Part model, mm, in its own coordinate system. A direction names the side the tool comes from. Coordinates: 2 decimals unless noted, no trailing zeros. Loops run counter-clockwise (first coordinate to the right, second up) from the corner with the lowest first, then second, coordinate; pieces in that order, holes last. Notation, with made-up numbers: (69, 70.25) -> (122, 70.25) arc R34 cw to (122, 108.25) -> close; hole circle Ø9 at (43.25, 68.5). An arc over 180 degrees is marked (long way). One line per item, written item: value. Start each with the question number.
from build123d import *

# Parameters (mm, degrees)
SKETCH1_W               = 16
SKETCH1_H               = 24
BOSS_EXTRUDE1_DEPTH     = 1
SKETCH2_W               = 12.3
SKETCH2_H               = 15.2
BOSS_EXTRUDE2_DEPTH     = 2.4
SKETCH3_R               = 0.3
CUT_EXTRUDE1_DEPTH      = 15.817557154
LPATTERN1_COUNT         = 8
LPATTERN1_PITCH         = 2
MIRROR1_COPY_1_SKETCH_R = 0.3
MIRROR1_COPY_1_DEPTH    = 15.817557154
MIRROR1_COPY_2_SKETCH_R = 0.3
MIRROR1_COPY_2_DEPTH    = 15.817557154
MIRROR1_COPY_3_SKETCH_R = 0.3
MIRROR1_COPY_3_DEPTH    = 15.817557154
MIRROR1_COPY_4_SKETCH_R = 0.3
MIRROR1_COPY_4_DEPTH    = 15.817557154
MIRROR1_COPY_5_SKETCH_R = 0.3
MIRROR1_COPY_5_DEPTH    = 15.817557154
MIRROR1_COPY_6_SKETCH_R = 0.3
MIRROR1_COPY_6_DEPTH    = 15.817557154
MIRROR1_COPY_7_SKETCH_R = 0.3
MIRROR1_COPY_7_DEPTH    = 15.817557154
SKETCH4_R               = 0.3
CUT_EXTRUDE2_DEPTH      = 15.817557154
LPATTERN2_COUNT         = 6
LPATTERN2_PITCH         = 2


with BuildPart() as part:
    # Sketch1 → Boss-Extrude1 (new body)
    with BuildSketch(Plane.XY):
        Rectangle(SKETCH1_W, SKETCH1_H)
    extrude(amount=BOSS_EXTRUDE1_DEPTH)

    # Sketch2 → Boss-Extrude2 (add)
    with BuildSketch(Plane.XY.offset(1)):
        with Locations((0, -3.1)):
            Rectangle(SKETCH2_W, SKETCH2_H)
    extrude(amount=BOSS_EXTRUDE2_DEPTH)

    # Sketch3 → Cut-Extrude1 (cut, through all)
    with BuildSketch(Plane(origin=(0, 0, 0), x_dir=(-1, 0, 0), z_dir=(0, 0, -1))):
        with Locations((8, -10.5)):
            Circle(SKETCH3_R)
    cut_extrude1 = extrude(amount=-CUT_EXTRUDE1_DEPTH, mode=Mode.SUBTRACT)

    # LPattern1: Cut-Extrude1 ×8
    with Locations(*[(0, i * LPATTERN1_PITCH, 0) for i in range(1, LPATTERN1_COUNT)]):
        add(cut_extrude1, mode=Mode.SUBTRACT)

    # Mirror1: Cut-Extrude1 across plane
    add(cut_extrude1.mirror(Plane(origin=(0, 0, 0), x_dir=(0, 0, 1), z_dir=(1, 0, 0))), mode=Mode.SUBTRACT)

    # Mirror1 copy 1 sketch → Mirror1 copy 1 (cut, through all)
    with BuildSketch(Plane(origin=(0, 2, 0), x_dir=(1, 0, 0), z_dir=(0, 0, -1))):
        with Locations((8, 10.5)):
            Circle(MIRROR1_COPY_1_SKETCH_R)
    extrude(amount=-MIRROR1_COPY_1_DEPTH, mode=Mode.SUBTRACT)

    # Mirror1 copy 2 sketch → Mirror1 copy 2 (cut, through all)
    with BuildSketch(Plane(origin=(0, 4, 0), x_dir=(1, 0, 0), z_dir=(0, 0, -1))):
        with Locations((8, 10.5)):
            Circle(MIRROR1_COPY_2_SKETCH_R)
    extrude(amount=-MIRROR1_COPY_2_DEPTH, mode=Mode.SUBTRACT)

    # Mirror1 copy 3 sketch → Mirror1 copy 3 (cut, through all)
    with BuildSketch(Plane(origin=(0, 6, 0), x_dir=(1, 0, 0), z_dir=(0, 0, -1))):
        with Locations((8, 10.5)):
            Circle(MIRROR1_COPY_3_SKETCH_R)
    extrude(amount=-MIRROR1_COPY_3_DEPTH, mode=Mode.SUBTRACT)

    # Mirror1 copy 4 sketch → Mirror1 copy 4 (cut, through all)
    with BuildSketch(Plane(origin=(0, 8, 0), x_dir=(1, 0, 0), z_dir=(0, 0, -1))):
        with Locations((8, 10.5)):
            Circle(MIRROR1_COPY_4_SKETCH_R)
    extrude(amount=-MIRROR1_COPY_4_DEPTH, mode=Mode.SUBTRACT)

    # Mirror1 copy 5 sketch → Mirror1 copy 5 (cut, through all)
    with BuildSketch(Plane(origin=(0, 10, 0), x_dir=(1, 0, 0), z_dir=(0, 0, -1))):
        with Locations((8, 10.5)):
            Circle(MIRROR1_COPY_5_SKETCH_R)
    extrude(amount=-MIRROR1_COPY_5_DEPTH, mode=Mode.SUBTRACT)

    # Mirror1 copy 6 sketch → Mirror1 copy 6 (cut, through all)
    with BuildSketch(Plane(origin=(0, 12, 0), x_dir=(1, 0, 0), z_dir=(0, 0, -1))):
        with Locations((8, 10.5)):
            Circle(MIRROR1_COPY_6_SKETCH_R)
    extrude(amount=-MIRROR1_COPY_6_DEPTH, mode=Mode.SUBTRACT)

    # Mirror1 copy 7 sketch → Mirror1 copy 7 (cut, through all)
    with BuildSketch(Plane(origin=(0, 14, 0), x_dir=(1, 0, 0), z_dir=(0, 0, -1))):
        with Locations((8, 10.5)):
            Circle(MIRROR1_COPY_7_SKETCH_R)
    extrude(amount=-MIRROR1_COPY_7_DEPTH, mode=Mode.SUBTRACT)

    # Sketch4 → Cut-Extrude2 (cut, through all)
    with BuildSketch(Plane(origin=(0, 0, 0), x_dir=(-1, 0, 0), z_dir=(0, 0, -1))):
        with Locations((5, -12)):
            Circle(SKETCH4_R)
    cut_extrude2 = extrude(amount=-CUT_EXTRUDE2_DEPTH, mode=Mode.SUBTRACT)

    # LPattern2: Cut-Extrude2 ×6
    with Locations(*[(i * LPATTERN2_PITCH, 0, 0) for i in range(1, LPATTERN2_COUNT)]):
        add(cut_extrude2, mode=Mode.SUBTRACT)


solid = part.part
1) Slice it at D-D (y = 7.5). Give the cut face in (x, z), then the cut area to 3 significant figures.
2) Probe line 1 (X direction, y = -1.75, z = 1.6); line 2 (Y direction, x = 0.5, z = 1.55); line 3 (Z direction, x = 4.25, y = 6.75). List the from-to ranges inside material, lowest first. Write a range as from..to.
3) Slice it at C-C (z = 1.35). Give the cut face in (x, y).
4) Pin check, flat tips, straight feed: pin 1 Ø1.2 at (x, z) = (-2, 2.5) entering from -Y; pin 2 Ø1.9 at (x, z) = (-1, 2.5) entering from +Y; pin 3 Ø2 at (y, z) = (7, 2.5) entering from +X; pin 4 Ø1.9 at (y, z) = (-3.5, 2.5) entering from -X. Stop position of each tip, or through.
5) Slice it at B-B (x = 2). Give the cut face in (y, z), then the cut area to 3 significant figures.
6) Slice it at A-A (y = -1.75). Give the cut face in (x, z).
7) Tool access for faces 1 (the flat face through (-6.15, -3, 2)), 2 (the flat face through (4, -12, 0.5)), 3 (the flat face through (-8, -3.5, 0.5)), 4 (the flat face through (0, -10.7, 2)), 5 (the flat face through (0, 4.5, 2)): list every direction of +Z, -Z, +X, -X, +Y, -Y with a clear straight run to the whole face (end or side of a thin tool).
Check sheet entries:
1. outline: (-8, 0) -> (8, 0) -> (8, 1) -> (-8, 1) -> close
1. area: 16.0 mm^2
2. line 1: x = -6.15..6.15
2. line 2: y = -10.7..4.5
2. line 3: z = 0..1
3. outline: (-6.15, -10.7) -> (6.15, -10.7) -> (6.15, 4.5) -> (-6.15, 4.5) -> close
4. pin 1: stops at y = -10.7
4. pin 2: stops at y = 4.5
4. pin 3: passes through
4. pin 4: stops at x = -6.15
5. outline: (-12, 0) -> (12, 0) -> (12, 1) -> (4.5, 1) -> (4.5, 3.4) -> (-10.7, 3.4) -> (-10.7, 1) -> (-12, 1) -> close
5. area: 60.5 mm^2
6. outline: (-8, 0) -> (8, 0) -> (8, 1) -> (6.15, 1) -> (6.15, 3.4) -> (-6.15, 3.4) -> (-6.15, 1) -> (-8, 1) -> close
7. face 1: +Z, -X, +Y, -Y
7. face 2: +Z, -Z, +X, -X, -Y
7. face 3: +Z, -Z, -X, +Y, -Y
7. face 4: +Z, +X, -X, -Y
7. face 5: +Z, +X, -X, +Y
